Here's how the part is built. I have some questions about the finished solid (model axes, mm). A direction names the side the tool comes from. Round coordinates to 2 decimals unless told otherwise and drop trailing zeros. Order: outer loops, then holes, each group sorted by start corner. A loop starts at its lowest first (then second) coordinate and runs counter-clockwise, first axis right, second up.
```python
from build123d import *

# Parameters (mm, degrees)
SKETCH1_W                                           = 50
SKETCH1_H                                           = 12
BOSS_EXTRUDE1_DEPTH                                 = 6
CBORE_FOR_M5_HEX_SOCKET_HEAD_CAP_SCREW1_D           = 5.5
CBORE_FOR_M5_HEX_SOCKET_HEAD_CAP_SCREW1_CBORE_D     = 10
CBORE_FOR_M5_HEX_SOCKET_HEAD_CAP_SCREW1_CBORE_DEPTH = 6


with BuildPart() as part:
    # Sketch1 → Boss-Extrude1 (new, symmetric)
    with BuildSketch(Plane(origin=(0, 0, 0), x_dir=(1, 0, 0), z_dir=(0, 1, 0))):
        with Locations((25, 6)):
            Rectangle(SKETCH1_W, SKETCH1_H)
    extrude(amount=BOSS_EXTRUDE1_DEPTH, both=True)

    # CBORE for M5 Hex Socket Head Cap Screw1 (through all)
    with Locations(Plane(origin=(0, 6, 0), x_dir=(1, 0, 0), z_dir=(0, 1, 0))):
        with Locations((42.5, 6), (7.5, 6)):
            CounterBoreHole(CBORE_FOR_M5_HEX_SOCKET_HEAD_CAP_SCREW1_D / 2, CBORE_FOR_M5_HEX_SOCKET_HEAD_CAP_SCREW1_CBORE_D / 2, CBORE_FOR_M5_HEX_SOCKET_HEAD_CAP_SCREW1_CBORE_DEPTH)


solid = part.part
```
1. If we section it at B-B, the plane x = 42.5: Write out the boundary of the cut face in (y, z).
Evaluation:
outline: (-6, -12) - (6, -12) - (6, -11) - (0, -11) - (0, -8.75) - (-6, -8.75) - close; (-6, -3.25) - (0, -3.25) - (0, -1) - (6, -1) - (6, 0) - (-6, 0) - close
2. If we section it at A-A, the plane z = -6: Write out the boundary of the cut face in (x, y), and give its area (3 significant figures).
Evaluation:
outline: (0, -6) - (4.75, -6) - (4.75, 0) - (2.5, 0) - (2.5, 6) - (0, 6) - close; (10.25, -6) - (39.75, -6) - (39.75, 0) - (37.5, 0) - (37.5, 6) - (12.5, 6) - (12.5, 0) - (10.25, 0) - close; (45.25, -6) - (50, -6) - (50, 6) - (47.5, 6) - (47.5, 0) - (45.25, 0) - close
area: 414 mm2
3. I need wall thicknesses on probe 1 along X at (y, z) = (-5.25, -5.75); probe 2 along X at (y, z) = (-2.25, -3.75); probe 3 along Z at (x, y) = (42.5, 2.6). Which ranges of each line are inside material? Lowest first, please.
Evaluation:
probe 1: x = 0 to 4.76, 10.24 to 39.76, 45.24 to 50
probe 2: x = 0 to 5.92, 9.08 to 40.92, 44.08 to 50
probe 3: z = -12 to -11, -1 to 0
4. On a 3-axis mill with a long thin cutter (end or side, diameter ignored), from which of +Z, -Z, +X, -X, +Y, -Y can I reach the whole of each face in a straight line? I mean faces 5 (the cylindrical face through (37.505, 3.042, -6.22)), 6 (the flat face through (25, 6, -6)). Say none if no direction works.
Evaluation:
face 5: +Y
face 6: +Z, -Z, +X, -X, +Y
5. I'm going to push flat-ended pins straight in: P1, Ø5, axis at x = 43.5, z = -6.5, coming from the +Y side; P2, Ø7, axis at x = 42.5, z = -6, coming from the -Y side. Where does each tip first touch, or does it pass through?
Evaluation:
P1: stops at y = 0
P2: stops at y = -6
6. If we section it at C-C, the plane y = 1.75: Write out the boundary of the cut face in (x, z), and give its area (3 significant figures).
Evaluation:
outline: (0, -12) - (50, -12) - (50, 0) - (0, 0) - close; hole circle Ø10 at (7.5, -6); hole circle Ø10 at (42.5, -6)
area: 443 mm2
7. If we section it at D-D, the plane x = 11.5: Write out the boundary of the cut face in (y, z), and give its area (3 significant figures).
Evaluation:
outline: (-6, -12) - (6, -12) - (6, -9) - (0, -9) - (0, -3) - (6, -3) - (6, 0) - (-6, 0) - close
area: 108 mm2
8. If we mould it in two halves opening along X, with no side actions, what happens to faces 1 (the flat face through (45, 0, -4)), 2 (the cylindrical face through (8.096, -3.042, -3.315)), 3 (the flat face through (50, 0, -6)), 4 (the flat face through (0, 0, -6))? For each: released by +X, released by -X, zero draft, split by the parting line, or undercut.
Evaluation:
face 1: undercut
face 2: undercut
face 3: released by +X
face 4: released by -X
